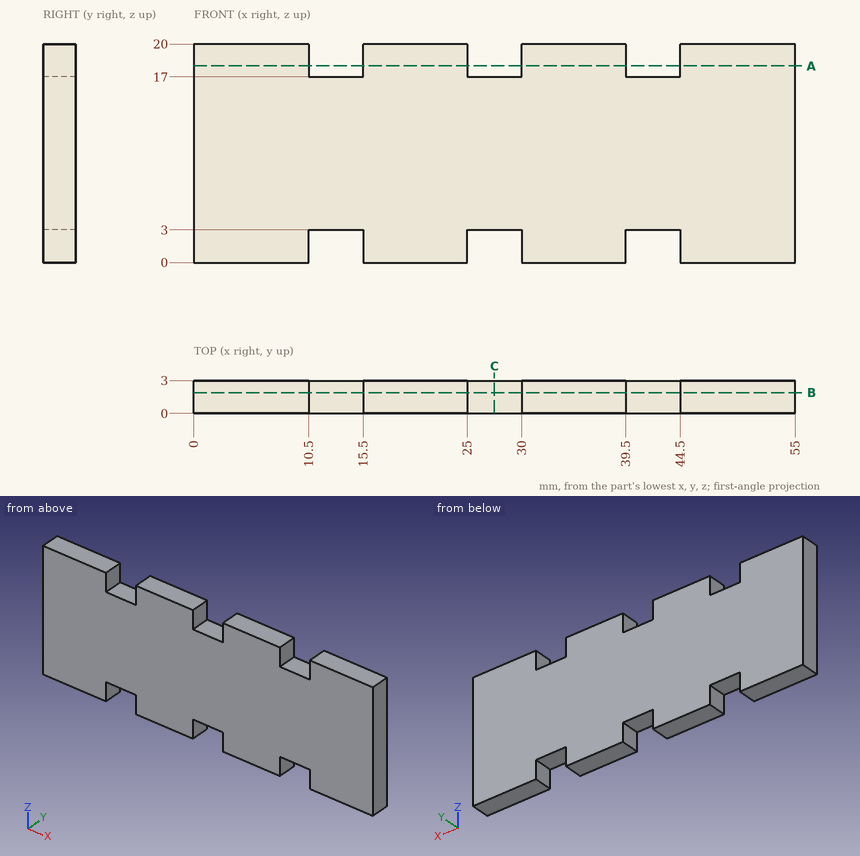
Design review of the part shown in the three views and the two pictorial views. Dimensions are in mm from the part's minimum x, y and z. Coordinates: 2 decimals unless noted, no trailing zeros. Order: outer loops, then holes, each group sorted by start corner. A loop starts at its lowest first (then second) coordinate and runs counter-clockwise, first axis right, second up. Notation, with made-up numbers: (-36, -13) - (-28, -13) arc R20 cw to (-28, 16) - close; hole circle Ø7 at (-14.75, -8.75). An arc over 180 degrees is marked (long way). Answer as CSV lines item,"result". Start each with the question number.
1) Insertion check: P1, Ø0.9, axis at x = 41.5, y = 2, coming from the -Z side; P2, Ø2, axis at x = 39.5, z = 5.5, coming from the -Y side; P3, Ø0.9, axis at x = 28, y = 2, coming from the +Z side. Each pin has a flat end and moves straight along its axis. Give the tip position at first contact, or say it passes through.
2) Add section B-B (y = 1.9). State the section outline as (x, z) points.
3) Add section A-A (z = 18). State the section outline as (x, y) points.
4) To check wall thickness, follow line 1 along X through (y, z) = (1, 18.25); line 2 along Z through (x, y) = (26.5, 0.55). State the ranges of each line that lie inside material, in increasing order. Write a range as [from, to].
5) Add section C-C (x = 27.5). State the section outline as (y, z) points.
Result:
1,P1,"z = 3"
1,P2,"y = 0"
1,P3,"z = 17"
2,outline,"(0, 0) - (10.5, 0) - (10.5, 3) - (15.5, 3) - (15.5, 0) - (25, 0) - (25, 3) - (30, 3) - (30, 0) - (39.5, 0) - (39.5, 3) - (44.5, 3) - (44.5, 0) - (55, 0) - (55, 20) - (44.5, 20) - (44.5, 17) - (39.5, 17) - (39.5, 20) - (30, 20) - (30, 17) - (25, 17) - (25, 20) - (15.5, 20) - (15.5, 17) - (10.5, 17) - (10.5, 20) - (0, 20) - close"
3,outline,"(0, 0) - (10.5, 0) - (10.5, 3) - (0, 3) - close; (15.5, 0) - (25, 0) - (25, 3) - (15.5, 3) - close; (30, 0) - (39.5, 0) - (39.5, 3) - (30, 3) - close; (44.5, 0) - (55, 0) - (55, 3) - (44.5, 3) - close"
4,line 1,"[0, 10.5], [15.5, 25], [30, 39.5], [44.5, 55]"
4,line 2,"[3, 17]"
5,outline,"(0, 3) - (3, 3) - (3, 17) - (0, 17) - close"
